Part model, mm, in its own coordinate system. Round coordinates to 2 decimals unless told otherwise and drop trailing zeros. Write each loop counter-clockwise with the first axis right and the second up, starting at its lowest first coordinate (ties: lowest second). Pieces come first, ordered by that corner, then holes. Notation, with made-up numbers: M 53.25,35.25 L 100.25,35.25 A16 ccw 100.25,40.25 Z; hole C 40,-37.75 d4. An arc over 180 degrees is marked long. Answer as a JSON object with one key per item and string values. Group by question number.
1. Drop flat-ended pins along their axis: pin 1 (13.5 mm diameter, centred on x = 0, y = 0, fed in from -Z); pin 2 (6 mm diameter, centred on x = 80.695, y = -23.57, fed in from +Z). Give the stop position or say it passes through.
2. Band-saw the part on A-A, the plane y = 0. Write the cut outline in (x, z) (3 decimals).
3. Band-saw the part on B-B, the plane x = 0. Write the cut outline in (y, z), plus the area to 3 significant figures.
4. Band-saw the part on C-C, the plane y = 23.57. Write the cut outline in (x, z) (3 decimals), plus the area to 3 significant figures.
5. Band-saw the part on D-D, the plane x = 34. Write the cut outline in (y, z), plus the area to 3 significant figures.
6. Drill centre lines: line 1 (X direction, y = -4.5, z = 0.8); line 2 (X direction, y = -15, z = 0.4); line 3 (X direction, y = -11.5, z = -0.3). Where is each one in solid material? Low to high. Write a range as from..to.
from build123d import *

# Parameters (mm, degrees)
SKETCH2_W               = 203.2
SKETCH2_H               = 88.9
SKETCH2_R               = 2.5
SKETCH2_R_2             = 19.15
BOSS_EXTRUDE1_DEPTH     = 1.27
SKETCH3_R               = 2.5
CUT_EXTRUDE1_DEPTH      = 111.92706658
CUT_EXTRUDE2_DEPTH      = 111.92706658
CUT_EXTRUDE2_DEPTH_BACK = 111.92706658
SKETCH4_R               = 7.5


with BuildPart() as part:
    # Sketch2 → Boss-Extrude1 (new, symmetric)
    with BuildSketch(Plane.XY):
        Rectangle(SKETCH2_W, SKETCH2_H)
        with Locations((-80.695, -23.57)):
            Circle(SKETCH2_R, mode=Mode.SUBTRACT)
        with Locations((-33.555, -23.57)):
            Circle(SKETCH2_R, mode=Mode.SUBTRACT)
        with Locations((-33.555, 23.57)):
            Circle(SKETCH2_R, mode=Mode.SUBTRACT)
        with Locations((-80.695, 23.57)):
            Circle(SKETCH2_R, mode=Mode.SUBTRACT)
        with Locations((33.555, 23.57)):
            Circle(SKETCH2_R, mode=Mode.SUBTRACT)
        with Locations((80.695, 23.57)):
            Circle(SKETCH2_R, mode=Mode.SUBTRACT)
        with Locations((33.555, -23.57)):
            Circle(SKETCH2_R, mode=Mode.SUBTRACT)
        with Locations((80.695, -23.57)):
            Circle(SKETCH2_R, mode=Mode.SUBTRACT)
        with Locations((-57.125, 0)):
            Circle(SKETCH2_R_2, mode=Mode.SUBTRACT)
        with Locations((57.125, 0)):
            Circle(SKETCH2_R_2, mode=Mode.SUBTRACT)
    extrude(amount=BOSS_EXTRUDE1_DEPTH, both=True)

    # Sketch3 → Cut-Extrude1 (cut, through all)
    with BuildSketch(Plane.XY.offset(1.27)):
        with Locations((-92.075, 34.925)):
            Circle(SKETCH3_R)
        with Locations((-92.075, -34.925)):
            Circle(SKETCH3_R)
        with Locations((92.075, -34.925)):
            Circle(SKETCH3_R)
        with Locations((92.075, 34.925)):
            Circle(SKETCH3_R)
    extrude(amount=-CUT_EXTRUDE1_DEPTH, mode=Mode.SUBTRACT)

    # Sketch4 → Cut-Extrude2 (cut, two sides: drawn at the far end of the back side and taken through both)
    with BuildSketch(Plane.XY.offset(1.27).offset(-CUT_EXTRUDE2_DEPTH_BACK)):
        Circle(SKETCH4_R)
    extrude(amount=CUT_EXTRUDE2_DEPTH + CUT_EXTRUDE2_DEPTH_BACK, mode=Mode.SUBTRACT)


solid = part.part
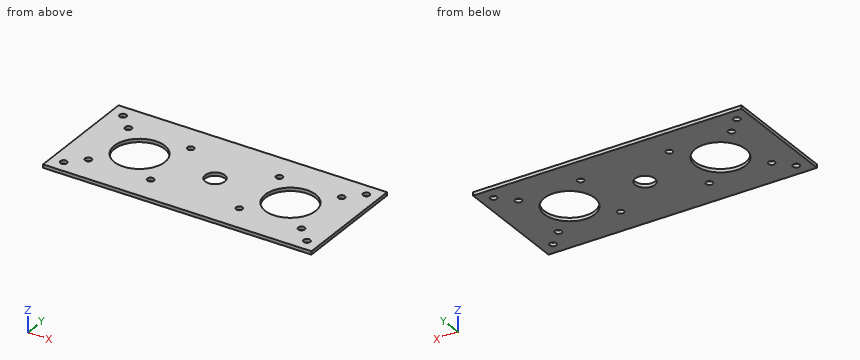
Worked answers:
{
 "1": {"pin 1": "passes through", "pin 2": "stops at z = 1.27"},
 "2": {"outline": "M -101.6,-1.27 L -76.275,-1.27 L -76.275,1.27 L -101.6,1.27 Z; M -37.975,-1.27 L -7.5,-1.27 L -7.5,1.27 L -37.975,1.27 Z; M 7.5,-1.27 L 37.975,-1.27 L 37.975,1.27 L 7.5,1.27 Z; M 76.275,-1.27 L 101.6,-1.27 L 101.6,1.27 L 76.275,1.27 Z"},
 "3": {"outline": "M -44.45,-1.27 L -7.5,-1.27 L -7.5,1.27 L -44.45,1.27 Z; M 7.5,-1.27 L 44.45,-1.27 L 44.45,1.27 L 7.5,1.27 Z", "area": "188 mm^2"},
 "4": {"outline": "M -101.6,-1.27 L -83.195,-1.27 L -83.195,1.27 L -101.6,1.27 Z; M -78.195,-1.27 L -36.055,-1.27 L -36.055,1.27 L -78.195,1.27 Z; M -31.055,-1.27 L 31.055,-1.27 L 31.055,1.27 L -31.055,1.27 Z; M 36.055,-1.27 L 78.195,-1.27 L 78.195,1.27 L 36.055,1.27 Z; M 83.195,-1.27 L 101.6,-1.27 L 101.6,1.27 L 83.195,1.27 Z", "area": "465 mm^2"},
 "5": {"outline": "M -44.45,-1.27 L -26.03,-1.27 L -26.03,1.27 L -44.45,1.27 Z; M -21.11,-1.27 L 21.11,-1.27 L 21.11,1.27 L -21.11,1.27 Z; M 26.03,-1.27 L 44.45,-1.27 L 44.45,1.27 L 26.03,1.27 Z", "area": "201 mm^2"},
 "6": {"line 1": "x = -101.6..-75.74, -38.51..-6, 6..38.51, 75.74..101.6", "line 2": "x = -101.6..-69.03, -45.22..45.22, 69.03..101.6", "line 3": "x = -101.6..-72.44, -41.81..41.81, 72.44..101.6"}
}
